Source: three-view drawing plus pictorial views. Frame: mm from the lowest corner of the part. Round coordinates to 2 decimals unless told otherwise and drop trailing zeros. Order: outer loops, then holes, each group sorted by start corner. A loop starts at its lowest first (then second) coordinate and runs counter-clockwise, first axis right, second up. Notation, with made-up numbers: (71, 47.5) -> (113, 47.5) arc R11 ccw to (113, 63.5) -> close; hole circle Ø7 at (57.5, -21.5). An arc over 180 degrees is marked (long way). Use a Markdown table: item, result.
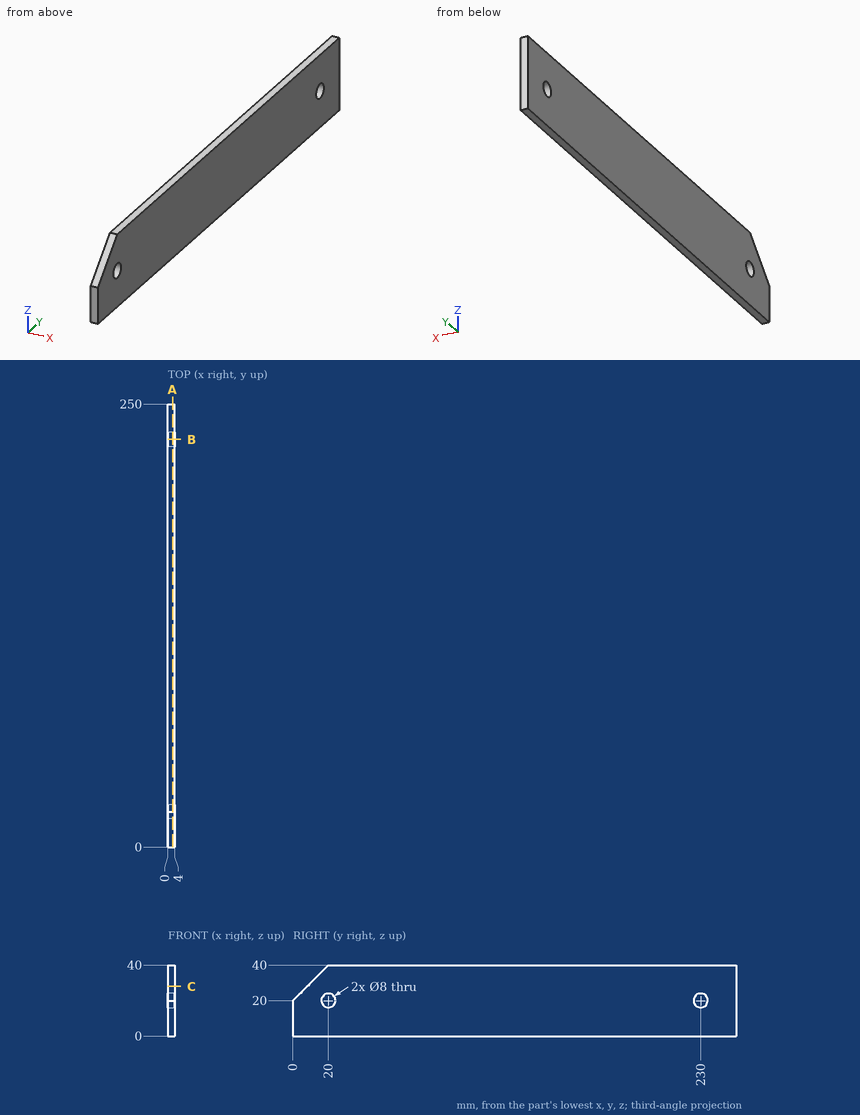
1) Line query: L1, parallel to Y at x = 1.4, z = 20; L2, parallel to Z at x = 2.7, y = 230; L3, parallel to Y at x = 1.9, z = 17. Output: solid intervals per line, ascending. Write a range as [from, to].
Results found:
| item | result |
|---|---|
| L1 | y = [0, 16], [24, 226], [234, 250] |
| L2 | z = [0, 16], [24, 40] |
| L3 | y = [0, 17.35], [22.65, 227.35], [232.65, 250] |
2) Cut plane B-B on y = 230. Return loops of the section in (x, z).
Results found:
| item | result |
|---|---|
| outline | (0, 0) -> (4, 0) -> (4, 16) -> (0, 16) -> close; (0, 24) -> (4, 24) -> (4, 40) -> (0, 40) -> close |
3) Cut plane C-C on z = 28. Return loops of the section in (x, y), and give its area (3 significant figures).
Results found:
| item | result |
|---|---|
| outline | (0, 8) -> (4, 8) -> (4, 250) -> (0, 250) -> close |
| area | 968 mm² |
4) Cut plane A-A on x = 2.7. Return loops of the section in (y, z), and give its area (3 significant figures).
Results found:
| item | result |
|---|---|
| outline | (0, 0) -> (250, 0) -> (250, 40) -> (20, 40) -> (0, 20) -> close; hole circle Ø8 at (20, 20); hole circle Ø8 at (230, 20) |
| area | 9,700 mm² |
